Verification items for the finished model (mm, model axes). A direction names the side the tool comes from. Give positions to 0.01 mm unless a question says otherwise; leave off trailing zeros. Write each loop counter-clockwise with the first axis right and the second up, starting at its lowest first coordinate (ties: lowest second). Pieces come first, ordered by that corner, then holes. Notation, with made-up numbers: M 68.25,-9.5 L 126.25,-9.5 A27 ccw 126.25,26.5 Z; hole C 57.25,31 d4. An arc over 180 degrees is marked long. Write item = value, one per line.
from build123d import *

# Parameters (mm, degrees)
F1_DEPTH = 86.5
F2_DEPTH = 45
F3_R     = 6.874276
F4_DEPTH = 100


with BuildPart() as f1:
    # F0 (on Front) → F1 (new body)
    with BuildSketch(Plane.XZ):
        with BuildLine():
            ThreePointArc((-26.142528, 15.448414), (-11.385953, 20.949011), (-5.185627, 35.42551))
            ThreePointArc((-5.185627, 35.42551), (-37.035985, 51.536655), (-31.142528, 16.333225))
            ThreePointArc((-31.142528, 16.333225), (-28.670722, 15.731498), (-26.142528, 15.448414))
        make_face()
    extrude(amount=F1_DEPTH)

    # F0 (on Front) → F2 (join)
    with BuildSketch(Plane.XZ):
        with BuildLine():
            ThreePointArc((-26.142528, 15.448414), (-28.670722, 15.731498), (-31.142528, 16.333225))
            Line((-31.142528, 16.333225), (-31.142528, -48.122729))
            Line((-31.142528, -48.122729), (-26.142528, -48.122729))
            Line((-26.142528, -48.122729), (-26.142528, 15.448414))
        make_face()
    extrude(amount=F2_DEPTH)

    # F3 (on face) → F4 (cut)
    with BuildSketch(Plane.XZ.offset(86.5)):
        with Locations((-25.185627, 35.42551)):
            Circle(F3_R)
    extrude(amount=-F4_DEPTH, mode=Mode.SUBTRACT)


solid = f1.part
1) Cross-section at C-C on z = -4. Record the boundary of the cut face in (x, y), plus the area to 3 significant figures.
From the geometry:
outline = M -31.14,-45 L -26.14,-45 L -26.14,0 L -31.14,0 Z
area = 225 mm^2
2) Cross-section at A-A on y = -25.5. Record the boundary of the cut face in (x, z), plus the area to 3 significant figures.
From the geometry:
outline = M -31.14,-48.12 L -26.14,-48.12 L -26.14,15.45 A20 ccw long -31.14,16.33 Z; hole C -25.19,35.43 d13.75
area = 1,430 mm^2
3) Cross-section at D-D on x = -10. Record the boundary of the cut face in (y, z), plus the area to 3 significant figures.
From the geometry:
outline = M -86.5,22.41 L 0,22.41 L 0,48.44 L -86.5,48.44 Z
area = 2,250 mm^2
4) Depth check by flat-ended pin: P1, Ø4, axis at x = -28, y = -67, coming from the -Z side; P2, Ø12, axis at x = -33.5, z = 1.5, coming from the -Y side; P3, Ø4, axis at y = -12.5, z = -23, coming from the +X side. Enter the tip coordinate at first touch or a pass-through.
From the geometry:
P1 = 15.44
P2 = -45
P3 = -26.14
5) Tool access check on faces 1 (the flat face through (-24, 0, 27)), 2 (the cylindrical face through (-28.71, -65.46, 15.74)). Record the directions out of +Z, -Z, +X, -X, +Y, -Y that give a thin tool (end or side, any length) a straight path to the whole face; none if there is none.
From the geometry:
face_1 = +Z, -Z, +X, -X, +Y
face_2 = -Z, -X, -Y
6) Cross-section at B-B on x = -22. Record the boundary of the cut face in (y, z), plus the area to 3 significant figures.
From the geometry:
outline = M -86.5,15.68 L 0,15.68 L 0,29.33 L -86.5,29.33 Z; M -86.5,41.52 L 0,41.52 L 0,55.17 L -86.5,55.17 Z
area = 2,360 mm^2
7) Material ranges on probe 1 along X at (y, z) = (-39, 5); probe 2 along Z at (x, y) = (-27, -34) (3 decimals); probe 3 along Z at (x, y) = (-28, -12), recorded low to high. Write a range as from..to.
From the geometry:
probe_1 = -31.14..-26.14
probe_2 = -48.123..28.795, 42.056..55.343
probe_3 = -48.12..29.15, 41.7..55.23
8) Draft check along X on faces 3 (the flat face through (-31.143, -22, -15)), 4 (the flat face through (-29, -45, -15)), 5 (the flat face through (-26.143, -22, -17)), 6 (the cylindrical face through (-21.49, -43.86, 41.22)). Enter one of: +X half, -X half, draft (parallel to the pull), parting line (faces both ways), or undercut.
From the geometry:
face_3 = -X half
face_4 = draft
face_5 = +X half
face_6 = undercut
